from build123d import *

# Parameters (mm, degrees)
BOSS_EXTRUDE1_DEPTH = 5.9436
SKETCH2_R           = 1.1303
SKETCH2_W           = 20.7
SKETCH2_H           = 41.3
CUT_EXTRUDE1_DEPTH  = 6.9436


with BuildPart() as part:
    # Sketch1 → Boss-Extrude1 (new body)
    with BuildSketch(Plane.XY):
        Polygon((6.35, 0), (6.35, -5.9436), (19.05, -5.9436), (19.05, 0), (31.75, 0), (31.75, -5.9436), (44.45, -5.9436), (44.45, 0), (50.8, 0), (50.8, 101.6), (0, 101.6), (0, 0), align=None)
    extrude(amount=BOSS_EXTRUDE1_DEPTH)

    # Sketch2 → Cut-Extrude1 (cut, through all)
    with BuildSketch(Plane.XY.offset(5.9436)):
        with Locations((20.4, 65.3)):
            Circle(SKETCH2_R)
        with Locations((30.4, 65.3)):
            Circle(SKETCH2_R)
        with Locations((20.4, 15)):
            Circle(SKETCH2_R)
        with Locations((30.4, 15)):
            Circle(SKETCH2_R)
        with Locations((25.4, 40.15)):
            Rectangle(SKETCH2_W, SKETCH2_H)
    extrude(amount=-CUT_EXTRUDE1_DEPTH, mode=Mode.SUBTRACT)


solid = part.part
Here's how the part is built. I have some questions about the finished solid (model axes, mm). A direction names the side the tool comes from. Give positions to 0.01 mm unless a question says otherwise; leave off trailing zeros. Order: outer loops, then holes, each group sorted by start corner. A loop starts at its lowest first (then second) coordinate and runs counter-clockwise, first axis right, second up. Notation, with made-up numbers: (-28, 76.5) -> (31, 76.5) arc R32 ccw to (31, 115.5) -> close; hole circle Ø6 at (81, 59). An arc over 180 degrees is marked (long way). One line per item, written item: value. Start each with the question number.
1. Imagine slicing it at A-A, the plane y = 15. List the corners of the cut face in (x, z) for me.
2. Will these pins go through, and if not, where does the flat tip stop? pin 1 Ø3 at (x, y) = (20.4, 65.3) entering from +Z; pin 2 Ø3 at (y, z) = (-2, 4.5) entering from -X; pin 3 Ø1 at (x, z) = (21.5, 1.5) entering from -Y; pin 4 Ø3 at (y, z) = (-2, 2) entering from +X.
3. Imagine slicing it at B-B, the plane x = 20.4. List the corners of the cut face in (y, z) for me, plus the area to 3 significant figures.
4. Imagine slicing it at D-D, the plane y = 52.5. List the corners of the cut face in (x, z) for me, plus the area to 3 significant figures.
5. For faces 1 (the face through (15.05, 40, 3)), 2 (the face through (25, 0, 3)), 3 (the face through (3, 0, 3)), which set-ups out of +Z, -Z, +X, -X, +Y, -Y let a thin tool reach every point of the face, with its end or its side?
6. We'd pull the mould along Y, two halves only. Please class faces 4 (the face through (26, 101.6, 3)), 5 (the face through (50.8, 50, 3)), 6 (the face through (30.25, 66.42, 3.01)): released by +Y, released by -Y, zero draft, split by the parting line, or undercut.
7. I need wall thicknesses on probe 1 along Y at (x, z) = (30.4, 3.3); probe 2 along X at (y, z) = (65.3, 4.35); probe 3 along Y at (x, z) = (34.5, 1.2). Which ranges of each line are inside material? Lowest first, please. Write a range as from..to.
8. Imagine slicing it at C-C, the plane z = 1.3. List the corners of the cut face in (x, y) for me, plus the area to 3 significant figures.
Values follow:
1. outline: (0, 0) -> (19.27, 0) -> (19.27, 5.94) -> (0, 5.94) -> close; (21.53, 0) -> (29.27, 0) -> (29.27, 5.94) -> (21.53, 5.94) -> close; (31.53, 0) -> (50.8, 0) -> (50.8, 5.94) -> (31.53, 5.94) -> close
2. pin 1: stops at z = 5.94
2. pin 2: stops at x = 6.35
2. pin 3: stops at y = 0
2. pin 4: stops at x = 44.45
3. outline: (0, 0) -> (13.87, 0) -> (13.87, 5.94) -> (0, 5.94) -> close; (16.13, 0) -> (19.5, 0) -> (19.5, 5.94) -> (16.13, 5.94) -> close; (60.8, 0) -> (64.17, 0) -> (64.17, 5.94) -> (60.8, 5.94) -> close; (66.43, 0) -> (101.6, 0) -> (101.6, 5.94) -> (66.43, 5.94) -> close
3. area: 332 mm2
4. outline: (0, 0) -> (15.05, 0) -> (15.05, 5.94) -> (0, 5.94) -> close; (35.75, 0) -> (50.8, 0) -> (50.8, 5.94) -> (35.75, 5.94) -> close
4. area: 179 mm2
5. face 1: +Z, -Z
5. face 2: +Z, -Z, -Y
5. face 3: +Z, -Z, -X, -Y
6. face 4: released by +Y
6. face 5: zero draft
6. face 6: undercut
7. probe 1: y = 0..13.87, 16.13..19.5, 60.8..64.17, 66.43..101.6
7. probe 2: x = 0..19.27, 21.53..29.27, 31.53..50.8
7. probe 3: y = -5.94..19.5, 60.8..101.6
8. outline: (0, 0) -> (6.35, 0) -> (6.35, -5.94) -> (19.05, -5.94) -> (19.05, 0) -> (31.75, 0) -> (31.75, -5.94) -> (44.45, -5.94) -> (44.45, 0) -> (50.8, 0) -> (50.8, 101.6) -> (0, 101.6) -> close; hole (15.05, 19.5) -> (35.75, 19.5) -> (35.75, 60.8) -> (15.05, 60.8) -> close; hole circle Ø2.26 at (20.4, 15); hole circle Ø2.26 at (20.4, 65.3); hole circle Ø2.26 at (30.4, 15); hole circle Ø2.26 at (30.4, 65.3)
8. area: 4,440 mm2
